Here's how the part is built. I have some questions about the finished solid (model axes, mm). A direction names the side the tool comes from. Give positions to 0.01 mm unless a question says otherwise; leave off trailing zeros. Write each loop counter-clockwise with the first axis right and the second up, starting at its lowest first coordinate (ties: lowest second). Pieces come first, ordered by that corner, then holes. Notation, with made-up numbers: M 33.5,-37.75 L 57.5,-37.75 A17 ccw 57.5,-15.75 Z; hole C 52.5,81.5 d5. An arc over 180 degrees is marked long. Answer as CSV lines item,"result". Start each with the question number.
Q1. Thinking about a two-plate mould opening in X: for faces 3 (the flat face through (22.5, 0, 4)), 4 (the flat face through (0, 0, 0)), 5 (the flat face through (0, 10, 6)), which applies, +X half, -X half, draft (parallel to the pull), parting line (faces both ways), or undercut?
Q2. Suppose I cut it at B-B (y = 20). Write out the boundary of the cut face in (x, z).
Q3. Suppose I cut it at A-A (z = 6). Write out the boundary of the cut face in (x, y).
Q4. Suppose I cut it at C-C (x = 14.5). Write out the boundary of the cut face in (y, z), then the cut area to 3 significant figures.
Q5. On a 3-axis mill with a long thin cutter (end or side, diameter ignored), from which of +Z, -Z, +X, -X, +Y, -Y can I reach the whole of each face in a straight line? I mean faces 1 (the flat face through (20, 0, 6)), 2 (the flat face through (0, -13, 8)). Say none if no direction works.
Q6. Suppose I cut it at D-D (x = -8). Write out the boundary of the cut face in (y, z).
Q7. For pin 1 (5 mm diameter, centred on x = 11, y = 0, fed in from -Z); pin 2 (8 mm diameter, centred on x = -14.5, y = 20, fed in from +Z), each with a flat end and sliding along its axis, tell me the tip position at first contact or that it passes through.
Q8. If I drill on line 1 along Y through (x, z) = (14.5, 6.7); line 2 along Y through (x, z) = (10, 4.75); line 3 along Y through (x, z) = (0.5, 4), over which ranges is the centre line in solid material (lowest first)?
```python
from build123d import *

# Parameters (mm, degrees)
SKETCH1_W           = 45
SKETCH1_H           = 60
BOSS_EXTRUDE1_DEPTH = 8
SKETCH2_R           = 5
SKETCH2_W           = 40
SKETCH2_H           = 20
CUT_EXTRUDE1_DEPTH  = 5


with BuildPart() as part:
    # Sketch1 → Boss-Extrude1 (new body)
    with BuildSketch(Plane.XY):
        Rectangle(SKETCH1_W, SKETCH1_H)
    extrude(amount=BOSS_EXTRUDE1_DEPTH)

    # Sketch2 → Cut-Extrude1 (cut)
    with BuildSketch(Plane.XY.offset(8)):
        with Locations((-14.5, 20)):
            Circle(SKETCH2_R)
        with Locations((14.5, 20)):
            Circle(SKETCH2_R)
        Rectangle(SKETCH2_W, SKETCH2_H)
    extrude(amount=-CUT_EXTRUDE1_DEPTH, mode=Mode.SUBTRACT)


solid = part.part
```
Resolved:
1,face 3,"+X half"
1,face 4,"draft"
1,face 5,"undercut"
2,outline,"M -22.5,0 L 22.5,0 L 22.5,8 L 19.5,8 L 19.5,3 L 9.5,3 L 9.5,8 L -9.5,8 L -9.5,3 L -19.5,3 L -19.5,8 L -22.5,8 Z"
3,outline,"M -22.5,-30 L 22.5,-30 L 22.5,30 L -22.5,30 Z; hole M -20,-10 L 20,-10 L 20,10 L -20,10 Z; hole C -14.5,20 d10; hole C 14.5,20 d10"
4,outline,"M -30,0 L 30,0 L 30,8 L 25,8 L 25,3 L 15,3 L 15,8 L 10,8 L 10,3 L -10,3 L -10,8 L -30,8 Z"
4,area,"330 mm^2"
5,face 1,"+Z"
5,face 2,"+Z, +X, -X, +Y, -Y"
6,outline,"M -30,0 L 30,0 L 30,8 L 10,8 L 10,3 L -10,3 L -10,8 L -30,8 Z"
7,pin 1,"z = 0"
7,pin 2,"z = 3"
8,line 1,"-30 to -10, 10 to 15, 25 to 30"
8,line 2,"-30 to -10, 10 to 17.82, 22.18 to 30"
8,line 3,"-30 to -10, 10 to 30"
